Check sheet for the modelled part. Datum: model origin and axes. Units: mm. A direction names the side the tool comes from. Give positions to 0.01 mm unless a question says otherwise; leave off trailing zeros. Loops run counter-clockwise (first coordinate to the right, second up) from the corner with the lowest first, then second, coordinate; pieces in that order, holes last. Notation, with made-up numbers: (-22, 38.5) - (-13, 38.5) arc R22 ccw to (-13, 76.5) - close; hole circle Ø8 at (69.5, 71). An arc over 180 degrees is marked (long way). Use CSV: the item, a comma, the result in double quotes.
from build123d import *

# Parameters (mm, degrees)
SKETCH1_R                = 25
SKETCH1_R_2              = 16
BOSS_EXTRUDE1_DEPTH      = 4
SKETCH2_R                = 1.6
CUT_EFFECTOR_HOLES_DEPTH = 36.580893749
SKETCH10_W               = 28
SKETCH10_H               = 4.287684823
CUT_EXTRUDE6_DEPTH       = 36.580893749
SKETCH3_W                = 28
SKETCH3_H                = 2
BOSS_FAN_EXTENSION_DEPTH = 4
BOSS_FAN_BOSS_DEPTH      = 4
CUT_FAN_SCREW_REACH      = 54.433
SKETCH5_R                = 2
CUT_FAN_HOLE_REACH       = 54.433
SKETCH6_R                = 18.5
FILLET1_R                = 2
CUT_EXTRUDE4_OUTLINE_R   = 1.6
CUT_EXTRUDE4_DEPTH       = 2
CUT_EXTRUDE4_DRAFT       = 10
CUT_EXTRUDE4_2_OUTLINE_R = 1.6
CUT_EXTRUDE4_2_DEPTH     = 2.484285969
CUT_EXTRUDE4_2_DRAFT     = 10
CUT_EXTRUDE4_3_OUTLINE_R = 1.6
CUT_EXTRUDE4_3_DEPTH     = 2
CUT_EXTRUDE4_3_DRAFT     = 10
CUT_EXTRUDE5_REACH       = 49.658
FILLET2_R                = 2
CUT_EXTRUDE7_DEPTH       = 2
CUT_EXTRUDE7_DRAFT       = -10
CUT_EXTRUDE7_2_DEPTH     = 2
CUT_EXTRUDE7_2_DRAFT     = -10


# Read off the part's stored shape, not the designer's step: Cut-Extrude4, Cut-Extrude7
with BuildPart() as part:
    # Sketch1 → Boss-Extrude1 (new body)
    with BuildSketch(Plane.XY):
        Circle(SKETCH1_R)
        Circle(SKETCH1_R_2, mode=Mode.SUBTRACT)
    extrude(amount=BOSS_EXTRUDE1_DEPTH)

    # Sketch2 → Cut-Effector Holes (cut, through all)
    with BuildSketch(Plane(origin=(0, 0, 0), x_dir=(-1, 0, 0), z_dir=(0, 0, -1))):
        with Locations((4.067203991, 18.133126642)):
            Circle(SKETCH2_R)
        with Locations((-13.670146326, -12.588865299)):
            Circle(SKETCH2_R)
        with Locations((16.454482672, -9.5)):
            Circle(SKETCH2_R)
    extrude(amount=-CUT_EFFECTOR_HOLES_DEPTH, mode=Mode.SUBTRACT)

    # Sketch10 → Cut-Extrude6 (cut, through all)
    with BuildSketch(Plane(origin=(0, 0, 0), x_dir=(-1, 0, 0), z_dir=(0, 0, -1))):
        with Locations((0, 22.856157589)):
            Rectangle(SKETCH10_W, SKETCH10_H)
    extrude(amount=-CUT_EXTRUDE6_DEPTH, mode=Mode.SUBTRACT)

    # Sketch3 → Boss-Fan Extension (add, through all)
    with BuildSketch(Plane.XY):
        with Locations((0, 21.712315177)):
            Rectangle(SKETCH3_W, SKETCH3_H)
    extrude(amount=BOSS_FAN_EXTENSION_DEPTH)

    # Sketch4 → Boss-Fan Boss (add)
    with BuildSketch(Plane(origin=(0, 11.356157589, -11.356157589), x_dir=(-1, 0, 0), z_dir=(0, 0.7071067811865464, -0.7071067811865488))):
        with BuildLine():
            Line((-20.5, 30.060032078), (-20.5, 36.060032078))
            Line((-20.5, 36.060032078), (20.5, 36.060032078))
            Line((20.5, 36.060032078), (20.5, 30.060032078))
            add(Edge.make_bspline(
                [(14, 18.888459203), (14, 26.407165397), (20.5, 22.786539918), (20.5, 30.060032078)],
                knots=[0, 0, 0, 0, 1, 1, 1, 1], degree=3))
            Line((14, 18.888459203), (14, 16.060032078))
            Line((14, 16.060032078), (-14, 16.060032078))
            Line((-14, 16.060032078), (-14, 18.888459203))
            add(Edge.make_bspline(
                [(-14, 18.888459203), (-14, 26.407165397), (-20.5, 22.786539918), (-20.5, 30.060032078)],
                knots=[0, 0, 0, 0, 1, 1, 1, 1], degree=3))
        make_face()
    extrude(amount=-BOSS_FAN_BOSS_DEPTH)

    # Sketch5 → Cut-Fan Screw (cut, up to next)
    with BuildSketch(Plane(origin=(0, 11.356157589, -11.356157589), x_dir=(1, 0, 0), z_dir=(0, 0.7071067811865466, -0.7071067811865485)), mode=Mode.PRIVATE) as cut_fan_screw_sk1:
        with Locations(Location((-16.5, -30.060032078, 0), (0, 0, 270))):
            Circle(SKETCH5_R)
    cut_fan_screw_tool1 = extrude(cut_fan_screw_sk1.sketch, amount=-CUT_FAN_SCREW_REACH, mode=Mode.PRIVATE) & part.part
    cut_fan_screw = cut_fan_screw_tool1.solids().sort_by_distance((-16.5, 32.61181, 9.899495))[0]
    add(cut_fan_screw, mode=Mode.SUBTRACT)

    # Mirror-Fan Screw: Cut-Fan Screw across plane
    add(cut_fan_screw.mirror(Plane(origin=(0, 0, 0), x_dir=(0, 0, 1), z_dir=(1, 0, 0))), mode=Mode.SUBTRACT)

    # Sketch6 → Cut-Fan Hole (cut, up to next)
    with BuildSketch(Plane(origin=(0, 11.356157589, -11.356157589), x_dir=(1, 0, 0), z_dir=(0, 0.7071067811865466, -0.7071067811865485)), mode=Mode.PRIVATE) as cut_fan_hole_sk1:
        with Locations((0, -46.560032078)):
            Circle(SKETCH6_R)
    cut_fan_hole_tool1 = extrude(cut_fan_hole_sk1.sketch, amount=-CUT_FAN_HOLE_REACH, mode=Mode.PRIVATE) & part.part
    add(cut_fan_hole_tool1.solids().sort_by_distance((0, 44.279072, 21.566757))[0], mode=Mode.SUBTRACT)

    # Fillet1
    fillet1_edges = [part.edges().sort_by_distance(p)[0] for p in [
        (20.5, 35.440237239, 15.556349186),
        (-20.5, 35.440237239, 15.556349186),
        (15.231546212, 35.440237239, 15.556349186),
        (-15.231546212, 35.440237239, 15.556349186),
    ]]
    fillet(fillet1_edges, radius=FILLET1_R)


with BuildPart() as cut_extrude4_tool:
    # Cut-Extrude4 outline → Cut-Extrude4 (with draft: the straight prism first)
    with BuildSketch(Plane(origin=(0, 0, 2), x_dir=(-1, 0, 0), z_dir=(0, 0, -1))):
        with BuildLine():
            ThreePointArc((-11.002045698, -11.617012975), (-11.701394046, -10.912258124), (-12.355684371, -10.165483939))
            Line((-12.355684371, -10.165483939), (-13.979106464, -9.42850504))
            Line((-13.979106464, -9.42850504), (-16.561578664, -11.276252498))
            Line((-16.561578664, -11.276252498), (-16.252618527, -14.436612757))
            Line((-16.252618527, -14.436612757), (-13.361186189, -15.749225558))
            Line((-13.361186189, -15.749225558), (-10.778713988, -13.901478101))
            Line((-10.778713988, -13.901478101), (-11.002045698, -11.617012975))
        make_face()
        with Locations((-13.670146326, -12.588865299)):
            Circle(CUT_EXTRUDE4_OUTLINE_R, mode=Mode.SUBTRACT)
    extrude(amount=-CUT_EXTRUDE4_DEPTH)
    # Cut-Extrude4: the draft: its side faces are tilted about the plane it starts from
    cut_extrude4_sides = [cut_extrude4_tool.faces().sort_by_distance(p)[0] for p in [
        (16.407098595, -12.856432627, 3),
        (14.806902358, -15.092919158, 3),
        (12.069950089, -14.825351829, 3),
        (10.890379843, -12.759245538, 3),
        (11.701394046, -10.912258124, 3),
        (13.167395417, -9.796994489, 3),
        (15.270342564, -10.352378769, 3),
        (15.270146326, -12.588865299, 3),
    ]]
    draft(cut_extrude4_sides, Plane(origin=(0, 0, 2), x_dir=(-1, 0, 0), z_dir=(0, 0, -1)), CUT_EXTRUDE4_DRAFT)


with BuildPart() as part_1:
    add(part.part)

    # Cut-Extrude4: cut by cut_extrude4_tool
    add(cut_extrude4_tool.part, mode=Mode.SUBTRACT)


with BuildPart() as cut_extrude4_2_tool:
    # Cut-Extrude4 2 outline → Cut-Extrude4 2 (with draft: the straight prism first)
    with BuildSketch(Plane(origin=(0, 0, 2), x_dir=(-1, 0, 0), z_dir=(0, 0, -1))):
        with BuildLine():
            ThreePointArc((2.378102624, 15.822282639), (3.371999625, 15.640639965), (4.352450444, 15.396628694))
            Line((4.352450444, 15.396628694), (6.010326315, 15.621631277))
            Line((6.010326315, 15.621631277), (7.21378394, 18.560172255))
            Line((7.21378394, 18.560172255), (5.270661616, 21.071667619))
            Line((5.270661616, 21.071667619), (2.124081667, 20.644622006))
            Line((2.124081667, 20.644622006), (0.920624042, 17.706081029))
            Line((0.920624042, 17.706081029), (2.378102624, 15.822282639))
        make_face()
        with Locations((4.067203991, 18.133126642)):
            Circle(CUT_EXTRUDE4_2_OUTLINE_R, mode=Mode.SUBTRACT)
    extrude(amount=-CUT_EXTRUDE4_2_DEPTH)
    # Cut-Extrude4 2: the draft: its side faces are tilted about the plane it starts from
    cut_extrude4_2_sides = [cut_extrude4_2_tool.faces().sort_by_distance(p)[0] for p in [
        (-6.242222778, 19.815919937, 3.242142985),
        (-3.697371642, 20.858144812, 3.242142985),
        (-1.522352855, 19.175351517, 3.242142985),
        (-1.649363333, 16.764181834, 3.242142985),
        (-3.371999625, 15.640639965, 3.242142985),
        (-5.18138838, 15.509129986, 3.242142985),
        (-6.612055127, 17.090901766, 3.242142985),
        (-2.467203991, 18.133126642, 3.242142985),
    ]]
    draft(cut_extrude4_2_sides, Plane(origin=(0, 0, 2), x_dir=(-1, 0, 0), z_dir=(0, 0, -1)), CUT_EXTRUDE4_2_DRAFT)


with BuildPart() as part_2:
    add(part_1.part)

    # Cut-Extrude4 2: cut by cut_extrude4_2_tool
    add(cut_extrude4_2_tool.part, mode=Mode.SUBTRACT)


with BuildPart() as cut_extrude4_3_tool:
    # Cut-Extrude4 3 outline → Cut-Extrude4 3 (with draft: the straight prism first)
    with BuildSketch(Plane(origin=(0, 0, 2), x_dir=(-1, 0, 0), z_dir=(0, 0, -1))):
        Polygon((18.042195912, -6.75), (14.866769432, -6.75), (13.279056191, -9.5), (14.866769432, -12.25), (18.042195912, -12.25), (19.629909152, -9.5), align=None)
        with Locations((16.454482672, -9.5)):
            Circle(CUT_EXTRUDE4_3_OUTLINE_R, mode=Mode.SUBTRACT)
    extrude(amount=-CUT_EXTRUDE4_3_DEPTH)
    # Cut-Extrude4 3: the draft: its side faces are tilted about the plane it starts from
    cut_extrude4_3_sides = [cut_extrude4_3_tool.faces().sort_by_distance(p)[0] for p in [
        (-16.454482672, -6.75, 3),
        (-14.072912812, -8.125, 3),
        (-14.072912812, -10.875, 3),
        (-16.454482672, -12.25, 3),
        (-18.836052532, -10.875, 3),
        (-18.836052532, -8.125, 3),
        (-14.854482672, -9.5, 3),
    ]]
    draft(cut_extrude4_3_sides, Plane(origin=(0, 0, 2), x_dir=(-1, 0, 0), z_dir=(0, 0, -1)), CUT_EXTRUDE4_3_DRAFT)


with BuildPart() as part_3:
    add(part_2.part)

    # Cut-Extrude4 3: cut by cut_extrude4_3_tool
    add(cut_extrude4_3_tool.part, mode=Mode.SUBTRACT)

    # Sketch8 → Cut-Extrude5 (cut, up to next)
    with BuildSketch(Plane(origin=(0, 0, 0), x_dir=(-1, 0, 0), z_dir=(0, 0, -1)), mode=Mode.PRIVATE) as cut_extrude5_sk1:
        with BuildLine():
            Line((9.279528916, -23.214011784), (5.602690803, -14.98698955))
            Line((5.602690803, -14.98698955), (7.428630962, -14.170936526))
            Line((7.428630962, -14.170936526), (11.105469075, -22.39795876))
            ThreePointArc((11.105469075, -22.39795876), (10.200662793, -22.824251983), (9.279528916, -23.214011784))
        make_face()
    cut_extrude5_tool1 = extrude(cut_extrude5_sk1.sketch, amount=-CUT_EXTRUDE5_REACH, mode=Mode.PRIVATE) & part_3.part
    add(cut_extrude5_tool1.solids().sort_by_distance((-8.356802, -18.698565, 0))[0], mode=Mode.SUBTRACT)

    # Fillet2
    fillet2_edges = [part_3.edges().sort_by_distance(p)[0] for p in [
        (-11.105469075, -22.39795876, 2),
        (-5.602690803, -14.98698955, 2),
        (-9.279528916, -23.214011784, 2),
        (-7.428630962, -14.170936526, 2),
    ]]
    fillet(fillet2_edges, radius=FILLET2_R)


with BuildPart() as cut_extrude7_tool:
    # Cut-Extrude7 outline → Cut-Extrude7 (with draft: the straight prism first)
    with BuildSketch(Plane(origin=(0, 9.941944026, -9.941944026), x_dir=(1, 0, 0), z_dir=(0, -0.7071067811865462, 0.7071067811865488))):
        Polygon((-13.8, 28.501186351), (-13.8, 31.618877805), (-16.5, 33.177723532), (-19.2, 31.618877805), (-19.2, 28.501186351), (-16.5, 26.942340625), align=None)
        with BuildLine():
            ThreePointArc((-16.5, 32.060032078), (-14.5, 30.060032078), (-16.5, 28.060032078))
            ThreePointArc((-16.5, 28.060032078), (-18.5, 30.060032078), (-16.5, 32.060032078))
        make_face(mode=Mode.SUBTRACT)
    extrude(amount=CUT_EXTRUDE7_DEPTH)
    # Cut-Extrude7: the draft: its side faces are tilted about the plane it starts from
    cut_extrude7_sides = [cut_extrude7_tool.faces().sort_by_distance(p)[0] for p in [
        (-13.8, 30.49048977, 12.02081528),
        (-16.5, 29.076276207, 10.606601718),
        (-17.85, 28.837084194, 10.367409704),
        (-19.2, 30.49048977, 12.02081528),
        (-17.85, 32.143895346, 13.674220857),
        (-15.15, 32.143895346, 13.674220857),
        (-15.15, 28.837084194, 10.367409704),
    ]]
    draft(cut_extrude7_sides, Plane(origin=(0, 9.941944026, -9.941944026), x_dir=(1, 0, 0), z_dir=(0, -0.7071067811865462, 0.7071067811865488)), CUT_EXTRUDE7_DRAFT)


with BuildPart() as part_4:
    add(part_3.part)

    # Cut-Extrude7: cut by cut_extrude7_tool
    add(cut_extrude7_tool.part, mode=Mode.SUBTRACT)


with BuildPart() as cut_extrude7_2_tool:
    # Cut-Extrude7 2 outline → Cut-Extrude7 2 (with draft: the straight prism first)
    with BuildSketch(Plane(origin=(0, 9.941944026, -9.941944026), x_dir=(1, 0, 0), z_dir=(0, -0.7071067811865462, 0.7071067811865488))):
        Polygon((19.2, 28.501186351), (19.2, 31.618877805), (16.5, 33.177723532), (13.8, 31.618877805), (13.8, 28.501186351), (16.5, 26.942340625), align=None)
        with BuildLine():
            ThreePointArc((16.5, 32.060032078), (18.5, 30.060032078), (16.5, 28.060032078))
            ThreePointArc((16.5, 28.060032078), (14.5, 30.060032078), (16.5, 32.060032078))
        make_face(mode=Mode.SUBTRACT)
    extrude(amount=CUT_EXTRUDE7_2_DEPTH)
    # Cut-Extrude7 2: the draft: its side faces are tilted about the plane it starts from
    cut_extrude7_2_sides = [cut_extrude7_2_tool.faces().sort_by_distance(p)[0] for p in [
        (19.2, 30.49048977, 12.02081528),
        (16.5, 29.076276207, 10.606601718),
        (15.15, 28.837084194, 10.367409704),
        (13.8, 30.49048977, 12.02081528),
        (15.15, 32.143895346, 13.674220857),
        (17.85, 32.143895346, 13.674220857),
        (17.85, 28.837084194, 10.367409704),
    ]]
    draft(cut_extrude7_2_sides, Plane(origin=(0, 9.941944026, -9.941944026), x_dir=(1, 0, 0), z_dir=(0, -0.7071067811865462, 0.7071067811865488)), CUT_EXTRUDE7_2_DRAFT)


with BuildPart() as part_5:
    add(part_4.part)

    # Cut-Extrude7 2: cut by cut_extrude7_2_tool
    add(cut_extrude7_2_tool.part, mode=Mode.SUBTRACT)


solid = part_5.part
1. Sectioned sample at A-A, the plane y = 0. Record the boundary of the cut face in (x, z).
Completed:
outline,"(-25, 0) - (-16, 0) - (-16, 4) - (-25, 4) - close; (16, 0) - (25, 0) - (25, 4) - (16, 4) - close"
2. Release check for a two-part mould opening along X. For faces 1 (the face through (-17, 0, 4)), 2 (the face through (-15.084, 28.732, 10.242)), 3 (the face through (-19.93, 34.995, 15.151)) record: released by +X, released by -X, zero draft, split by the parting line, or undercut.
Completed:
face 1,"zero draft"
face 2,"undercut"
face 3,"released by -X"
3. Sectioned sample at B-B, the plane x = -11. Record the boundary of the cut face in (y, z), and give its area (3 significant figures).
Completed:
outline,"(-21.3, 0) - (-11.62, 0) - (-11.62, 4) - (-21.3, 4) - close; (11.62, 0) - (22.71, 0) - (33.76, 11.05) - (30.93, 13.88) - (21.06, 4) - (11.62, 4) - close"
area,"139 mm²"
4. Go/stop test with flat-tipped pins: pin 1 Ø2 at (x, z) = (-10.5, 5) entering from +Y; pin 2 Ø8 at (x, z) = (20, 2) entering from -Y; pin 3 Ø17 at (x, y) = (11.5, 0.5) entering from +Z. Record where each tip stops, or that it passes through.
Completed:
pin 1,"stops at y = 28.71"
pin 2,"stops at y = -19.21"
pin 3,"stops at z = 4"
5. Set-up check for faces 4 (the face through (-15.04, 32.25, 13.76)), 5 (the face through (-25, 0, 2)), 6 (the face through (-19.374, 30.518, 12.028)), 7 (the face through (15, -14, 2)), 8 (the face through (-8.065, -14.405, 2.028)): record each of +Z, -Z, +X, -X, +Y, -Y from which the full face is reachable in a straight line by a thin tool's end or side.
Completed:
face 4,"-Y"
face 5,"+Z, -Z, -X"
face 6,"none"
face 7,"+Z"
face 8,"+Z, -Z"
6. Sectioned sample at C-C, the plane y = -19. Record the boundary of the cut face in (x, z), and give its area (3 significant figures).
Completed:
outline,"(-16.25, 0) - (-9.59, 0) - (-9.59, 4) - (-16.25, 4) - close; (-7.4, 0) - (16.25, 0) - (16.25, 4) - (-7.4, 4) - close"
area,"121 mm²"
7. Scan lines: line 1 along X through (y, z) = (0, 3); line 2 along Z through (x, y) = (10.5, 13); line 3 along Y through (x, z) = (0, 1.1). Record each from-to range of solid material in increasing order.
Completed:
line 1,"x = -25 to -16, 16 to 25"
line 2,"z = 0 to 4"
line 3,"y = -25 to -16, 16 to 23.81"
